```python
from build123d import *

# Parameters (mm, degrees)
ESQUISSE1_W             = 73
ESQUISSE1_H             = 35
ESQUISSE1_R             = 1.75
BOSS_EXTRU_1_DEPTH      = 2
BOSS_EXTRU_2_DEPTH      = 10
ESQUISSE3_W             = 26.5
ESQUISSE3_H             = 35
BOSS_EXTRU_3_DEPTH      = 2
ESQUISSE4_W             = 19.5
ESQUISSE4_H             = 35
BOSS_EXTRU_4_DEPTH      = 3.5
CONG_1_R                = 2
ESQUISSE5_W             = 6
ESQUISSE5_H             = 4
ENL_V_MAT_EXTRU_1_DEPTH = 35
CONG_2_R                = 0.5


with BuildPart() as part:
    # Esquisse1 → Boss.-Extru.1 (new body)
    with BuildSketch(Plane.XY):
        Rectangle(ESQUISSE1_W, ESQUISSE1_H)
        with Locations((-26.5, 10)):
            Circle(ESQUISSE1_R, mode=Mode.SUBTRACT)
        with Locations((-26.5, -10)):
            Circle(ESQUISSE1_R, mode=Mode.SUBTRACT)
        with Locations(Location((26.5, -10, 0), (0, 0, 180))):
            Circle(ESQUISSE1_R, mode=Mode.SUBTRACT)
        with Locations(Location((26.5, 10, 0), (0, 0, 180))):
            Circle(ESQUISSE1_R, mode=Mode.SUBTRACT)
    extrude(amount=-BOSS_EXTRU_1_DEPTH)

    # Esquisse2 → Boss.-Extru.2 (add)
    with BuildSketch(Plane(origin=(0, 0, -2), x_dir=(-1, 0, 0), z_dir=(0, 0, -1))):
        with BuildLine():
            Line((6, 15.5), (6, 9.5))
            ThreePointArc((6, 9.5), (4, 7.5), (2, 9.5))
            Line((2, 9.5), (2, 15.5))
            ThreePointArc((2, 15.5), (4, 17.5), (6, 15.5))
        make_face()
        with BuildLine():
            Line((6, -15.5), (6, -9.5))
            ThreePointArc((6, -9.5), (4, -7.5), (2, -9.5))
            Line((2, -9.5), (2, -15.5))
            ThreePointArc((2, -15.5), (4, -17.5), (6, -15.5))
        make_face()
        Polygon((10, 17.5), (10, 5.5), (2, 2.5), (2, -2.5), (10, -5.5), (10, -17.5), (21.5, -17.5), (21.5, 17.5), align=None)
    extrude(amount=BOSS_EXTRU_2_DEPTH)

    # Esquisse3 → Boss.-Extru.3 (add)
    with BuildSketch(Plane(origin=(0, 0, -12), x_dir=(-1, 0, 0), z_dir=(0, 0, -1))):
        with Locations((15.25, 0)):
            Rectangle(ESQUISSE3_W, ESQUISSE3_H)
    extrude(amount=BOSS_EXTRU_3_DEPTH)

    # Esquisse4 → Boss.-Extru.4 (add)
    with BuildSketch(Plane(origin=(0, 0, -2), x_dir=(-1, 0, 0), z_dir=(0, 0, -1))):
        with Locations((11.75, 0)):
            Rectangle(ESQUISSE4_W, ESQUISSE4_H)
    extrude(amount=BOSS_EXTRU_4_DEPTH)

    # Congé1
    cong_1_edges = [part.edges().sort_by_distance(p)[0] for p in [
        (-2, 17.5, -3.75),
        (-2, -17.5, -3.75),
        (-10, 17.5, -8.75),
        (-10, 5.5, -8.75),
        (-2, 2.5, -8.75),
        (-2, -2.5, -8.75),
        (-10, -5.5, -8.75),
        (-10, -17.5, -8.75),
        (-2, 17.5, -13),
        (-2, -17.5, -13),
        (-28.5, -17.5, -13),
        (-28.5, 17.5, -13),
    ]]
    fillet(cong_1_edges, radius=CONG_1_R - 0.0001)  # a hair under: the kernel refuses the full size

    # Esquisse5 → Enlèv. mat.-Extru.1 (cut)
    with BuildSketch(Plane(origin=(0, 17.5, 0), x_dir=(1, 0, 0), z_dir=(0, 1, 0))):
        with Locations((-15.5, 12)):
            Rectangle(ESQUISSE5_W, ESQUISSE5_H)
    extrude(amount=-ENL_V_MAT_EXTRU_1_DEPTH, mode=Mode.SUBTRACT)

    # Congé2
    cong_2_edges = [part.edges().sort_by_distance(p)[0] for p in [
        (-28.5, 0, -14),
        (-8.24995, -17.5, -14),
        (-2, 0, -14),
        (-22.50005, 17.5, -14),
        (-2.585757148, 16.914242852, -14),
        (-2.585757148, -16.914242852, -14),
        (-27.914242852, 16.914242852, -14),
        (-27.914242852, -16.914242852, -14),
        (-22.50005, -17.5, -14),
        (-8.24995, 17.5, -14),
        (-12.5, 17.5, -12),
        (-18.5, 17.5, -12),
        (-15.5, 17.5, -10),
        (-18.5, 0, -14),
        (-18.5, -17.5, -12),
        (-18.5, 0, -10),
        (-15.5, -17.5, -10),
        (-12.5, 0, -10),
        (-12.5, -17.5, -12),
        (-12.5, 0, -14),
    ]]
    fillet(cong_2_edges, radius=CONG_2_R)


solid = part.part
```
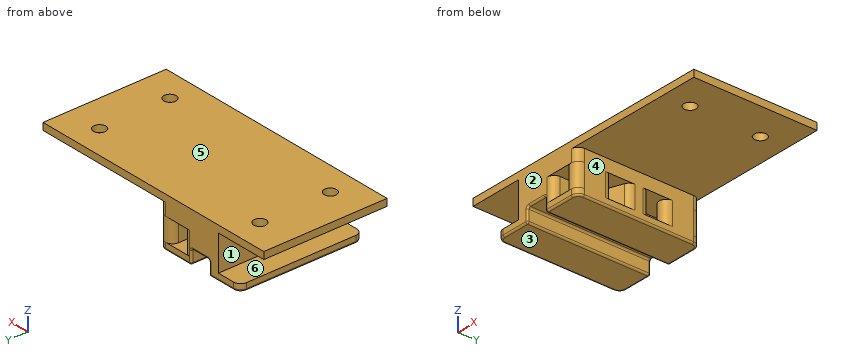
Verification items for the finished model (mm, model axes). Face numbers are marked on the shaded views. A direction names the side the tool comes from. Give positions to 0.01 mm unless a question says otherwise; leave off trailing zeros. Order: outer loops, then holes, each group sorted by start corner. A loop starts at its lowest first (then second) coordinate and runs counter-clockwise, first axis right, second up. Notation, with made-up numbers: M -13.5,75 L 1.5,75 A33 ccw 1.5,112 Z; hole C -19,-7 d11. An arc over 180 degrees is marked long. Return JSON: item names as keys, results as strings. Group by question number.
1) Access from +Z, -Z, +X, -X, +Y, -Y to the whole of each face (thin tool, end or side, straight path). Record for the marked faces 1 and 2.
2) Scan lines: line 1 (Y direction, x = 26.5, z = -1.3); line 2 (X direction, y = 13.5, z = -11.75); line 3 (Z direction, x = -9.5, y = 10). Record each from-to range of solid material in increasing order.
3) Go/stop test with flat-tipped pins: pin 1 Ø5.5 at (x, y) = (-15.5, 1) entering from -Z; pin 2 Ø3 at (y, z) = (-10.5, -7) entering from +X; pin 3 Ø2.5 at (y, z) = (0.5, -12.5) entering from -X. Record where each tip stops, or that it passes through.
4) Section check D-D on x = -32. Record the cut outline in (y, z), and give its area (3 significant figures).
5) Section check C-C on z = -7.5. Record the cut outline in (x, y), and give its area (3 significant figures).
6) Section check A-A on z = -11.25. Give the number of separate pieces and of enclosed holes in the cut face, and give its area (3 significant figures).
7) Mould release check, pull along Z, two halves, no side actions. Record for the marked faces 3, 4, 5 and 6: pulls with the +Z half, pulls with the -Z half, needs draft (parallel to the pull), parting line crosses it, or undercut.
8) Section check B-B on y = 12.5. Record the cut outline in (x, z).
Answer block:
{
 "1": {"face 1": "-X, +Y, -Y", "face 2": "+Z, -Z, +X, -X, -Y"},
 "2": {"line 1": "y = -17.5 to -11.75, -8.25 to 8.25, 11.75 to 17.5", "line 2": "x = -21.5 to -18.5, -12.5 to -10, -6 to -2", "line 3": "z = -14 to -12, -5.5 to 0"},
 "3": {"pin 1": "stops at z = -10.07", "pin 2": "stops at x = -2", "pin 3": "stops at x = -28.5"},
 "4": {"outline": "M -17.5,-2 L 17.5,-2 L 17.5,0 L -17.5,0 Z", "area": "70.0 mm^2"},
 "5": {"outline": "M -21.5,-17.5 L -12,-17.5 A2 ccw -10,-15.5 L -10,-6.89 A2 cw -8.7,-5.01 L -3.3,-2.99 A2 ccw -2,-1.11 L -2,1.11 A2 ccw -3.3,2.99 L -8.7,5.01 A2 cw -10,6.89 L -10,15.5 A2 ccw -12,17.5 L -21.5,17.5 Z; M -6,-15.5 A2 ccw -2,-15.5 L -2,-9.5 A2 ccw -6,-9.5 Z; M -6,9.5 A2 ccw -2,9.5 L -2,15.5 A2 ccw -6,15.5 Z", "area": "538 mm^2"},
 "6": {"separate pieces": "4", "enclosed holes": "0", "area": "328 mm^2"},
 "7": {"face 3": "pulls with the -Z half", "face 4": "needs draft", "face 5": "pulls with the +Z half", "face 6": "undercut"},
 "8": {"outline": "M -36.5,-2 L -21.5,-2 L -21.5,-12 L -28.5,-12 L -28.5,-13.5 A0.5 ccw -28,-14 L -19,-14 A0.5 ccw -18.5,-13.5 L -18.5,-10.5 A0.5 cw -18,-10 L -13,-10 A0.5 cw -12.5,-10.5 L -12.5,-13.5 A0.5 ccw -12,-14 L -2.5,-14 A0.5 ccw -2,-13.5 L -2,-2 L 36.5,-2 L 36.5,0 L -36.5,0 Z; hole M -10,-12 L -6,-12 L -6,-5.5 L -10,-5.5 Z"}
}
